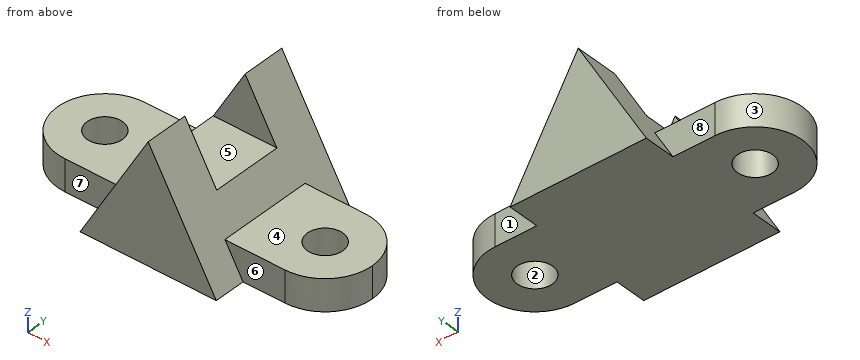
from build123d import *

# Parameters (mm, degrees)
F0_R     = 7.14375
F1_DEPTH = 12.7
F3_DEPTH = 31.75
F5_DEPTH = 25.4


with BuildPart() as f1:
    # F0 (on Top) → F1 (new body)
    with BuildSketch(Plane.XY):
        with BuildLine():
            Line((-25.4, 0), (0, 0))
            Line((0, 0), (25.4, 0))
            ThreePointArc((25.4, 0), (30.9796158184, 13.4703841816), (44.45, 19.05))
            Line((44.45, 19.05), (-44.45, 19.05))
            ThreePointArc((-44.45, 19.05), (-30.9796158184, 13.4703841816), (-25.4, 0))
        make_face()
        with BuildLine():
            Line((25.4, 0), (0, 0))
            Line((0, 0), (-25.4, 0))
            ThreePointArc((-25.4, 0), (-30.9796158184, -13.4703841816), (-44.45, -19.05))
            Line((-44.45, -19.05), (44.45, -19.05))
            ThreePointArc((44.45, -19.05), (30.9796158184, -13.4703841816), (25.4, 0))
        make_face()
        with BuildLine():
            ThreePointArc((44.45, 19.05), (30.9796158184, 13.4703841816), (25.4, 0))
            ThreePointArc((25.4, 0), (30.9796158184, -13.4703841816), (44.45, -19.05))
            ThreePointArc((44.45, -19.05), (57.9203841816, -13.4703841816), (63.5, 0))
            ThreePointArc((63.5, 0), (57.9203841816, 13.4703841816), (44.45, 19.05))
        make_face()
        with BuildLine():
            ThreePointArc((51.59375, 0), (44.45, -7.14375), (37.30625, 0))
            ThreePointArc((37.30625, 0), (44.45, 7.14375), (51.59375, 0))
        make_face(mode=Mode.SUBTRACT)
        with BuildLine():
            ThreePointArc((-44.45, -19.05), (-30.9796158184, -13.4703841816), (-25.4, 0))
            ThreePointArc((-25.4, 0), (-30.9796158184, 13.4703841816), (-44.45, 19.05))
            ThreePointArc((-44.45, 19.05), (-63.5, 0), (-44.45, -19.05))
        make_face()
        with Locations((-44.45, 0)):
            Circle(F0_R, mode=Mode.SUBTRACT)
    extrude(amount=F1_DEPTH)

    # F2 (on Front) → F3 (join, symmetric)
    with BuildSketch(Plane.XZ):
        Polygon((27.4963065702, 0), (0, 47.625), (-27.4963065702, 0), align=None)
    extrude(amount=F3_DEPTH, both=True)

    # F4 (on Right) → F5 (cut, symmetric)
    with BuildSketch(Plane.YZ):
        Polygon((14.2875, 47.625), (0, 47.625), (-14.2875, 47.625), (-14.2875, 25.4), (14.2875, 25.4), align=None)
    extrude(amount=F5_DEPTH, both=True, mode=Mode.SUBTRACT)


solid = f1.part
Geometry check sheet. Reference: the model listing, model coordinates, mm. Face numbers are marked on the shaded views. A direction names the side the tool comes from. Round coordinates to 2 decimals unless told otherwise and drop trailing zeros. Write each loop counter-clockwise with the first axis right and the second up, starting at its lowest first coordinate (ties: lowest second). Pieces come first, ordered by that corner, then holes. Notation, with made-up numbers: (40, 58.5) -> (82, 58.5) arc R14 cw to (82, 83.5) -> close; hole circle Ø4 at (87.5, 22). An arc over 180 degrees is marked (long way). One line per item, written item: value. Start each with the question number.
(1) Access from +Z, -Z, +X, -X, +Y, -Y to the whole of each face (thin tool, end or side, straight path). Record for the marked faces 4, 5, 6, 7 and 8.
(2) Cross-section at A-A, the plane z = 43. Record the cut outline in (x, y).
(3) Go/stop test with flat-tipped pins: pin 1 Ø14 at (x, z) = (36, 3.5) entering from -Y; pin 2 Ø4 at (x, z) = (36.5, 6.5) entering from +Y; pin 3 Ø1.5 at (y, z) = (-10.5, 16) entering from -X; pin 4 Ø6 at (x, y) = (-43.5, 15) entering from -Z. Record where each tip stops, or that it passes through.
(4) Cross-section at C-C, the plane z = 4. Record the cut outline in (x, y).
(5) Cross-section at D-D, the plane y = 26.5. Record the cut outline in (x, z) (3 decimals), and give its area (3 significant figures).
(6) Scan lines: line 1 (Y direction, x = -44.45, z = 7.25); line 2 (Y direction, x = -1, z = 37.5); line 3 (Z direction, x = 57, y = 4.5). Record each from-to range of solid material in increasing order. Write a range as [from, to].
(7) Draft check along X on the marked faces 1, 2 and 3. Enter one of: +X half, -X half, draft (parallel to the pull), parting line (faces both ways), or undercut.
(8) Cross-section at B-B, the plane x = 46. Record the cut outline in (y, z).
Answer:
1. face 4: +Z, +X, +Y, -Y
1. face 5: +Z, +X, -X
1. face 6: +Z, +X, -Y
1. face 7: +Z, -X, -Y
1. face 8: +Z, -X, +Y
2. outline: (-2.67, -31.75) -> (2.67, -31.75) -> (2.67, -14.29) -> (-2.67, -14.29) -> close; (-2.67, 14.29) -> (2.67, 14.29) -> (2.67, 31.75) -> (-2.67, 31.75) -> close
3. pin 1: y = -19.05
3. pin 2: y = 19.05
3. pin 3: x = -18.69
3. pin 4: z = 0
4. outline: (-44.45, -19.05) -> (-25.19, -19.05) -> (-25.19, -31.75) -> (25.19, -31.75) -> (25.19, -19.05) -> (44.45, -19.05) arc R19.05 ccw to (44.45, 19.05) -> (25.19, 19.05) -> (25.19, 31.75) -> (-25.19, 31.75) -> (-25.19, 19.05) -> (-44.45, 19.05) arc R19.05 ccw to start; hole circle Ø14.29 at (-44.45, 0); hole circle Ø14.29 at (44.45, 0)
5. outline: (-27.496, 0) -> (27.496, 0) -> (0, 47.625) -> close
5. area: 1,310 mm²
6. line 1: [-19.05, -7.14], [7.14, 19.05]
6. line 2: [-31.75, -14.29], [14.29, 31.75]
6. line 3: [0, 12.7]
7. face 1: draft
7. face 2: undercut
7. face 3: -X half
8. outline: (-18.99, 0) -> (-6.97, 0) -> (-6.97, 12.7) -> (-18.99, 12.7) -> close; (6.97, 0) -> (18.99, 0) -> (18.99, 12.7) -> (6.97, 12.7) -> close
